```python
from build123d import *

# Parameters (mm, degrees)
F0_R     = 1.190625
F0_R_2   = 1.5875
F1_DEPTH = 1.5875
F2_SIZE  = 0.762


with BuildPart() as f1:
    # F0 (on Front) → F1 (new body, symmetric)
    with BuildSketch(Plane.XZ):
        with BuildLine():
            Line((-4.19507, -3.443071), (-4.164685, -4.719849))
            ThreePointArc((-4.164685, -4.719849), (6.575626, 10.980695), (-5.78257, -3.480852))
            Line((-5.78257, -3.480852), (-4.19507, -3.443071))
        make_face()
        with Locations((7.395771, 0.439879)):
            Circle(F0_R, mode=Mode.SUBTRACT)
        with Locations((0.784385, 3.418477)):
            Circle(F0_R_2, mode=Mode.SUBTRACT)
    extrude(amount=F1_DEPTH, both=True)

    # F2
    f2_edges = [f1.edges().sort_by_distance(p)[0] for p in [
        (6.205146, -1.5875, 0.439879),
    ]]
    chamfer(f2_edges, length=F2_SIZE)


solid = f1.part
```
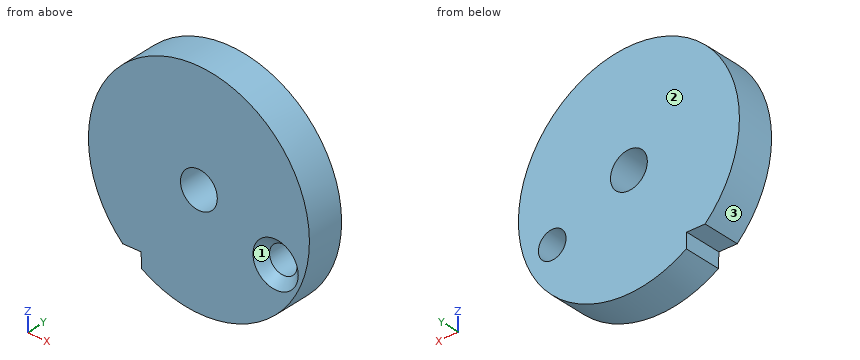
Geometry: final body of the model. Coordinates: model frame, mm. Face numbers are marked on the shaded views. Round coordinates to 2 decimals unless told otherwise and drop trailing zeros. Loops run counter-clockwise (first coordinate to the right, second up) from the corner with the lowest first, then second, coordinate; pieces in that order, holes last. Notation, with made-up numbers: (10.25, -17.75) -> (54.25, -17.75) arc R12 cw to (54.25, 2.25) -> close; hole circle Ø1 at (-27, -27). An arc over 180 degrees is marked (long way). Write each question's results on one line, items separated by ' | '.
Item 1: Pin query (flat end, axial travel): pin 1 Ø5 at (x, z) = (0.78, 3.42) entering from -Y. Return the tip coordinate at first contact, or that it passes through.
Answers below:
pin 1: stops at y = -1.59
Item 2: Cut plane C-C on y = 0.45. State how many separate pieces and enclosed holes the cut face has, and give its area (3 significant figures).
Answers below:
separate pieces: 1 | enclosed holes: 2 | area: 272 mm²
Item 3: Cut plane D-D on z = 8.25. Return the cut outline in (x, y), and give its area (3 significant figures).
Answers below:
outline: (-7.42, -1.59) -> (8.99, -1.59) -> (8.99, 1.59) -> (-7.42, 1.59) -> close | area: 52.1 mm²
Item 4: Pull-direction query (Z, two-part tool) for the marked faces 1, 2 and 3; classes: pulls with the +Z half, pulls with the -Z half, needs draft (parallel to the pull), parting line crosses it, or undercut.
Answers below:
face 1: undercut | face 2: needs draft | face 3: parting line crosses it
Item 5: Cut plane B-B on x = 1.5. Return the cut outline in (y, z).
Answers below:
outline: (-1.59, -6.08) -> (1.59, -6.08) -> (1.59, 2) -> (-1.59, 2) -> close; (-1.59, 4.84) -> (1.59, 4.84) -> (1.59, 12.92) -> (-1.59, 12.92) -> close
Item 6: Cut plane A-A on z = 4.25. Return the cut outline in (x, y), and give its area (3 significant figures).
Answers below:
outline: (-8.7, -1.59) -> (-0.57, -1.59) -> (-0.57, 1.59) -> (-8.7, 1.59) -> close; (2.14, -1.59) -> (10.27, -1.59) -> (10.27, 1.59) -> (2.14, 1.59) -> close | area: 51.7 mm²
Item 7: Line query: probe 1 along X at (y, z) = (0.5, -0.25); probe 2 along X at (y, z) = (0.6, 3); probe 3 along Z at (x, y) = (-0.5, -0.95). Output: solid intervals per line, ascending. Write a range as [from, to].
Answers below:
probe 1: x = [-8.01, 6.43], [8.37, 9.57] | probe 2: x = [-8.73, -0.75], [2.32, 10.3] | probe 3: z = [-6.02, 2.49], [4.35, 12.86]
